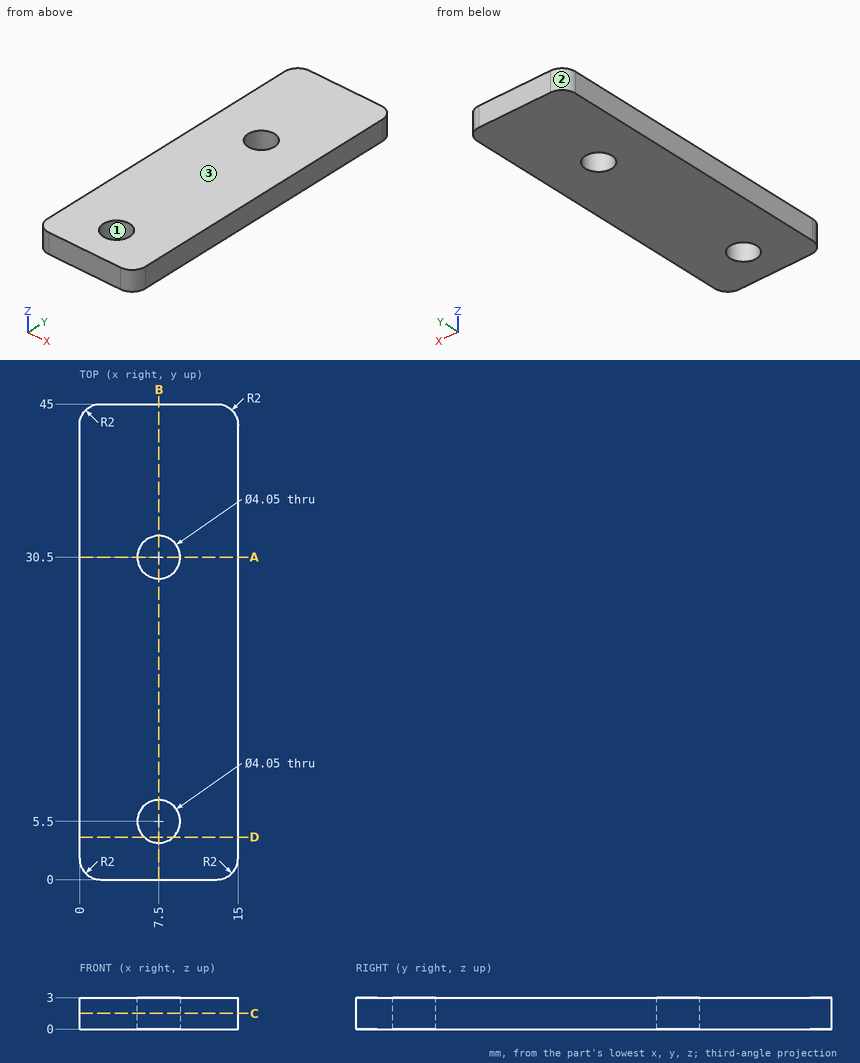
For this review, use the dimensioned drawing (mm, ordinates from the lowest corner) and the shaded views. Round coordinates to 2 decimals unless told otherwise and drop trailing zeros. Write each loop counter-clockwise with the first axis right and the second up, starting at its lowest first coordinate (ties: lowest second). Pieces come first, ordered by that corner, then holes. Notation, with made-up numbers: M -34,43.5 L -15,43.5 A26 cw -15,80.5 Z; hole C 83,-10.75 d9. An arc over 180 degrees is marked long. Write item = value, one per line. Start each with the question number.
(1) The part is to be moulded in two halves that separate along X. For the marked faces 1, 2 and 3, say which applies: +X half, -X half, draft (parallel to the pull), parting line (faces both ways), or undercut.
(2) Clearance check with a flat-ended pin moving along its axis: pin 1 Ø3 at (x, y) = (7.5, 30.5) entering from +Z. State where the tip first meets the part, or that it passes through.
(3) For line 1 along Y through (x, z) = (7.5, 2.25) (3 decimals); line 2 along Y through (x, z) = (9.25, 2.5); line 3 along Y through (x, z) = (13.5, 2.4), list the stretches that pass through material, from the lowest coordinate up.
(4) We need section B-B (x = 7.5). Give the boundary of the cut face in (y, z) (3 decimals), then the cut area to 3 significant figures.
(5) We need section C-C (z = 1.5). Give the boundary of the cut face in (x, y) (3 decimals), then the cut area to 3 significant figures.
(6) We need section D-D (y = 4). Give the boundary of the cut face in (x, z).
(7) We need section A-A (y = 30.5). Give the boundary of the cut face in (x, z) (3 decimals), then the cut area to 4 significant figures.
Results found:
q1.face_1 = undercut
q1.face_2 = -X half
q1.face_3 = draft
q2.pin_1 = through
q3.line_1 = 0 to 3.475, 7.525 to 28.475, 32.525 to 45
q3.line_2 = 0 to 4.48, 6.52 to 29.48, 31.52 to 45
q3.line_3 = 0.06 to 44.94
q4.outline = M 0,0 L 3.475,0 L 3.475,3 L 0,3 Z; M 7.525,0 L 28.475,0 L 28.475,3 L 7.525,3 Z; M 32.525,0 L 45,0 L 45,3 L 32.525,3 Z
q4.area = 111 mm²
q5.outline = M 0,2 A2 ccw 2,0 L 13,0 A2 ccw 15,2 L 15,43 A2 ccw 13,45 L 2,45 A2 ccw 0,43 Z; hole C 7.5,5.5 d4.05; hole C 7.5,30.5 d4.05
q5.area = 646 mm²
q6.outline = M 0,0 L 6.14,0 L 6.14,3 L 0,3 Z; M 8.86,0 L 15,0 L 15,3 L 8.86,3 Z
q7.outline = M 0,0 L 5.475,0 L 5.475,3 L 0,3 Z; M 9.525,0 L 15,0 L 15,3 L 9.525,3 Z
q7.area = 32.85 mm²
